Source: CAD feature listing. Evaluate the final solid. Frame: model axes, mm. A direction names the side the tool comes from. Round coordinates to 2 decimals unless told otherwise and drop trailing zeros. Loops run counter-clockwise (first coordinate to the right, second up) from the corner with the lowest first, then second, coordinate; pieces in that order, holes last.
Item 1: Section query B-B on y = -7.5. Return loops of the section in (x, z).
Item 2: Access query for faces 5 (the flat face through (14, 20.7, 0)), 6 (the flat face through (-8.67, 0.03, 4.98)). Directions: +Z, -Z, +X, -X, +Y, -Y. A direction counts if a zero-diameter tool reaches every point of the face in a straight line with its end or side. Return the directions, or none.
Item 3: Pull-direction query (Y, two-part tool) for faces 1 (the cylindrical face through (12.5, -0.8, 5.1)), 2 (the flat face through (8.65, 20.03, 5.02)), 3 (the flat face through (7, -20.7, -12)), 4 (the cylindrical face through (-4.798, 23.235, 10.676)); classes: released by +Y, released by -Y, zero draft, split by the parting line, or undercut.
Item 4: First-contact query: P1, Ø4.5, axis at x = 0, y = 0, coming from the -Z side; P2, Ø1, axis at x = 7.5, y = 1.5, coming from the -Z side; P3, Ø2, axis at y = -17, z = 12, coming from the -X side; P4, Ø3.5, axis at x = -6.75, z = -11.69, coming from the +Y side. Flat tips, straight axial feed; report the tip coordinate or a pass-through.
Item 5: Section query A-A on y = 20. Return loops of the section in (x, z), then the cut area to 3 significant figures.
Item 6: Ray query, L1, parallel to X at y = 25.05, z = 0; L2, parallel to X at y = 19.5, z = 4; L3, parallel to Z at x = -12, y = 0.5. Return the intervals inside material, ascending.
```python
from build123d import *

# Parameters (mm, degrees)
CYLINDER011_R               = 2
CYLINDER011_DEPTH           = 10
CYLINDER010_R               = 2
CYLINDER010_DEPTH           = 10
CYLINDER009_R               = 2
CYLINDER009_DEPTH           = 10
CYLINDER009_PLACEMENT_ANGLE = -8.000003
CYLINDER008_R               = 2
CYLINDER008_DEPTH           = 10
CYLINDER007_R               = 2
CYLINDER007_DEPTH           = 10
CYLINDER006_R               = 2
CYLINDER006_DEPTH           = 10
CYLINDER005_R               = 2
CYLINDER005_DEPTH           = 10
CYLINDER004_R               = 2
CYLINDER004_DEPTH           = 10
CYLINDER003_R               = 2
CYLINDER003_DEPTH           = 10
CYLINDER002_R               = 2
CYLINDER002_DEPTH           = 10
CYLINDER001_R               = 2
CYLINDER001_DEPTH           = 10
CYLINDER001_PLACEMENT_ANGLE = 9.999992
CYLINDER_R                  = 2
CYLINDER_DEPTH              = 10
SKETCH001_R                 = 2.2
POCKET_DEPTH                = 5
SKETCH002_R                 = 2.2
POCKET001_DEPTH             = 5
CUT_PLACEMENT_ANGLE         = 119.999977
CUT001_PLACEMENT_ANGLE      = 119.999977
CUT003_PLACEMENT_ANGLE      = 119.999977
CUT004_PLACEMENT_ANGLE      = 119.999977
CUT006_PLACEMENT_ANGLE      = 119.999977
CUT007_PLACEMENT_ANGLE      = 119.999977
CUT008_PLACEMENT_ANGLE      = 60.000023
CUT009_PLACEMENT_ANGLE      = 119.999977
CUT010_PLACEMENT_ANGLE      = 119.999977


with BuildPart() as cylinder011:
    # Cylinder011 → Cylinder011 (new body)
    with BuildSketch(Plane.XY.offset(10)):
        Circle(CYLINDER011_R)
    extrude(amount=CYLINDER011_DEPTH)


with BuildPart() as cylinder010:
    # Cylinder010 → Cylinder010 (new body)
    with BuildSketch(Plane.XY.offset(10)):
        Circle(CYLINDER010_R)
    extrude(amount=CYLINDER010_DEPTH)


with BuildPart() as cylinder009:
    # Cylinder009 → Cylinder009 (new body)
    with BuildSketch(Plane.XY):
        Circle(CYLINDER009_R)
    extrude(amount=CYLINDER009_DEPTH)


with BuildPart() as cylinder009_1:
    # Cylinder009 placement: moved
    add(cylinder009.part.moved(Location((0, 0, 10))).rotate(Axis((0, 0, 10), (0, 0, 1)), CYLINDER009_PLACEMENT_ANGLE))


with BuildPart() as cylinder008:
    # Cylinder008 → Cylinder008 (new body)
    with BuildSketch(Plane(origin=(0, -20, 10), x_dir=(1, 0, 0), z_dir=(0, 0, 1))):
        Circle(CYLINDER008_R)
    extrude(amount=CYLINDER008_DEPTH)


with BuildPart() as cylinder007:
    # Cylinder007 → Cylinder007 (new body)
    with BuildSketch(Plane(origin=(0, -20, 10), x_dir=(1, 0, 0), z_dir=(0, 0, 1))):
        Circle(CYLINDER007_R)
    extrude(amount=CYLINDER007_DEPTH)


with BuildPart() as cylinder006:
    # Cylinder006 → Cylinder006 (new body)
    with BuildSketch(Plane(origin=(0, -20, 10), x_dir=(1, 0, 0), z_dir=(0, 0, 1))):
        Circle(CYLINDER006_R)
    extrude(amount=CYLINDER006_DEPTH)


with BuildPart() as cylinder005:
    # Cylinder005 → Cylinder005 (new body)
    with BuildSketch(Plane(origin=(0, 20, 10), x_dir=(1, 0, 0), z_dir=(0, 0, 1))):
        Circle(CYLINDER005_R)
    extrude(amount=CYLINDER005_DEPTH)


with BuildPart() as cylinder004:
    # Cylinder004 → Cylinder004 (new body)
    with BuildSketch(Plane(origin=(0, 20, 10), x_dir=(1, 0, 0), z_dir=(0, 0, 1))):
        Circle(CYLINDER004_R)
    extrude(amount=CYLINDER004_DEPTH)


with BuildPart() as cylinder003:
    # Cylinder003 → Cylinder003 (new body)
    with BuildSketch(Plane(origin=(0, 20, 10), x_dir=(1, 0, 0), z_dir=(0, 0, 1))):
        Circle(CYLINDER003_R)
    extrude(amount=CYLINDER003_DEPTH)


with BuildPart() as cylinder002:
    # Cylinder002 → Cylinder002 (new body)
    with BuildSketch(Plane.XY.offset(10)):
        Circle(CYLINDER002_R)
    extrude(amount=CYLINDER002_DEPTH)


with BuildPart() as cylinder001:
    # Cylinder001 → Cylinder001 (new body)
    with BuildSketch(Plane.XY):
        Circle(CYLINDER001_R)
    extrude(amount=CYLINDER001_DEPTH)


with BuildPart() as cylinder001_1:
    # Cylinder001 placement: moved
    add(cylinder001.part.moved(Location((0, 0, 10))).rotate(Axis((0, 0, 10), (0, 0, 1)), CYLINDER001_PLACEMENT_ANGLE))


with BuildPart() as cylinder:
    # Cylinder → Cylinder (new body)
    with BuildSketch(Plane.XY.offset(10)):
        Circle(CYLINDER_R)
    extrude(amount=CYLINDER_DEPTH)


with BuildPart() as cut011:
    # Sketch → Revolution (revolve)
    with BuildSketch(Plane.YZ):
        Polygon((-24.5, 8), (-24.5, 9), (-25, 9.01746), (-24.5, 10.31746), (-25.7, 10.31746), (-25.7, 16.9), (25.7, 16.9), (25.7, 10.31746), (24.5, 10.31746), (25, 9.01746), (24.5, 9), (24.5, 8), align=None)
    revolve(axis=Axis((0, 0, 0), (0, 1, 0)))

    # Sketch001 → Pocket (cut)
    with BuildSketch(Plane(origin=(0, -25.7, 0), x_dir=(0, 0, -1), z_dir=(0, -1, 0))):
        with Locations((-11.691342, 6.750002)):
            Circle(SKETCH001_R)
        with Locations((-11.691342, -6.750002)):
            Circle(SKETCH001_R)
        with Locations((0, -13.5)):
            Circle(SKETCH001_R)
        with Locations((11.691342, -6.750002)):
            Circle(SKETCH001_R)
        with Locations((11.691342, 6.750002)):
            Circle(SKETCH001_R)
        with Locations((0, 13.5)):
            Circle(SKETCH001_R)
    extrude(amount=-POCKET_DEPTH, mode=Mode.SUBTRACT)

    # Sketch002 → Pocket001 (cut)
    with BuildSketch(Plane.ZX.offset(25.7)):
        with Locations((0, 13.5)):
            Circle(SKETCH002_R)
        with Locations((11.691342, 6.750002)):
            Circle(SKETCH002_R)
        with Locations((11.691342, -6.750002)):
            Circle(SKETCH002_R)
        with Locations((0, -13.5)):
            Circle(SKETCH002_R)
        with Locations((-11.691342, -6.750002)):
            Circle(SKETCH002_R)
        with Locations((-11.691342, 6.750002)):
            Circle(SKETCH002_R)
    extrude(amount=-POCKET001_DEPTH, mode=Mode.SUBTRACT)

    # Cut: cut Cylinder
    add(cylinder.part, mode=Mode.SUBTRACT)


with BuildPart() as cut011_1:
    # Cut placement: moved
    add(cut011.part.rotate(Axis((0, 0, 0), (0, 1, 0)), CUT_PLACEMENT_ANGLE))

    # Cut001: cut Cylinder001
    add(cylinder001_1.part, mode=Mode.SUBTRACT)


with BuildPart() as cut011_2:
    # Cut001 placement: moved
    add(cut011_1.part.rotate(Axis((0, 0, 0), (0, 1, 0)), CUT001_PLACEMENT_ANGLE))

    # Cut002: cut Cylinder002
    add(cylinder002.part, mode=Mode.SUBTRACT)

    # Cut003: cut Cylinder003
    add(cylinder003.part, mode=Mode.SUBTRACT)


with BuildPart() as cut011_3:
    # Cut003 placement: moved
    add(cut011_2.part.rotate(Axis((0, 0, 0), (0, 1, 0)), CUT003_PLACEMENT_ANGLE))

    # Cut004: cut Cylinder004
    add(cylinder004.part, mode=Mode.SUBTRACT)


with BuildPart() as cut011_4:
    # Cut004 placement: moved
    add(cut011_3.part.rotate(Axis((0, 0, 0), (0, 1, 0)), CUT004_PLACEMENT_ANGLE))

    # Cut005: cut Cylinder005
    add(cylinder005.part, mode=Mode.SUBTRACT)

    # Cut006: cut Cylinder006
    add(cylinder006.part, mode=Mode.SUBTRACT)


with BuildPart() as cut011_5:
    # Cut006 placement: moved
    add(cut011_4.part.rotate(Axis((0, 0, 0), (0, 1, 0)), CUT006_PLACEMENT_ANGLE))

    # Cut007: cut Cylinder007
    add(cylinder007.part, mode=Mode.SUBTRACT)


with BuildPart() as cut011_6:
    # Cut007 placement: moved
    add(cut011_5.part.rotate(Axis((0, 0, 0), (0, 1, 0)), CUT007_PLACEMENT_ANGLE))

    # Cut008: cut Cylinder008
    add(cylinder008.part, mode=Mode.SUBTRACT)


with BuildPart() as cut011_7:
    # Cut008 placement: moved
    add(cut011_6.part.rotate(Axis((0, 0, 0), (0, 1, 0)), CUT008_PLACEMENT_ANGLE))

    # Cut009: cut Cylinder009
    add(cylinder009_1.part, mode=Mode.SUBTRACT)


with BuildPart() as cut011_8:
    # Cut009 placement: moved
    add(cut011_7.part.rotate(Axis((0, 0, 0), (0, 1, 0)), CUT009_PLACEMENT_ANGLE))

    # Cut010: cut Cylinder010
    add(cylinder010.part, mode=Mode.SUBTRACT)


with BuildPart() as cut011_9:
    # Cut010 placement: moved
    add(cut011_8.part.rotate(Axis((0, 0, 0), (0, 1, 0)), CUT010_PLACEMENT_ANGLE))

    # Cut011: cut Cylinder011
    add(cylinder011.part, mode=Mode.SUBTRACT)


solid = cut011_9.part
```
Data:
1. outline: circle Ø33.8 at (0, 0); hole circle Ø16 at (0, 0)
2. face 5: +Y
2. face 6: none
3. face 1: undercut
3. face 2: undercut
3. face 3: released by -Y
3. face 4: zero draft
4. P1: stops at z = -16.9
4. P2: stops at z = -15.38
4. P3: stops at x = -12.83
4. P4: stops at y = 20.7
5. outline: (-15.53, 6.66) arc R16.9 ccw to (-2, -16.78) - (-2, -10) - (2, -10) - (2, -16.78) arc R16.9 ccw to (15.53, 6.66) - (9.66, 3.27) - (7.66, 6.73) - (13.53, 10.12) arc R16.9 ccw to (-13.53, 10.12) - (-7.66, 6.73) - (-9.66, 3.27) - close; hole circle Ø16 at (0, 0)
5. area: 614 mm2
6. L1: x = -16.9 to -15.7, -11.3 to -10.32, 10.32 to 11.3, 15.7 to 16.9
6. L2: x = -16.42 to -10.8, -9.24 to -6.93, 6.93 to 9.24, 10.8 to 16.42
6. L3: z = -11.9 to -9.16, -4.69 to 4.69, 9.16 to 11.9
